Can you work these out from the model? Positions are in its coordinate system, mm. A direction names the side the tool comes from. Give positions to 0.01 mm unless a question says otherwise; leave off trailing zeros. Loops run counter-clockwise (first coordinate to the right, second up) from the corner with the lowest first, then second, coordinate; pieces in that order, holes last. Notation, with made-up numbers: (19.5, 38) -> (42.5, 38) arc R22 cw to (42.5, 69) -> close; hole circle Ø8 at (-11, 56). An arc over 180 degrees is marked (long way). Return JSON: item names as keys, results as strings. Group by question number.
Q1. Will these pins go through, and if not, where does the flat tip stop? pin 1 (0.6 mm diameter, centred on y = -11, z = 4, fed in from -X); pin 2 (0.6 mm diameter, centred on y = -11, z = 11, fed in from +X).
Q2. Suppose I cut it at A-A, the plane z = 6.5. Please give me the cut outline in (x, y), and give its area (3 significant figures).
Q3. Which directions (+Z, -Z, +X, -X, +Y, -Y) give clear straight access to the entire face, cutting with the end or side of a thin tool? Please do faces 1 (the flat face through (-11.498, -11, 7)), 2 (the flat face through (-5, -10, 8)), 3 (the flat face through (-1.4, 25, 7.4)).
Q4. I need wall thicknesses on line 1 along Y through (x, z) = (-15.75, 8.25); line 2 along Y through (x, z) = (-11.75, 10.75); line 3 along X through (y, z) = (8, 1). Which ranges of each line are inside material? Lowest first, please. Write a range as [from, to].
```python
from build123d import *

# Parameters (mm, degrees)
F0_W         = 20
F0_H         = 15
F1_DEPTH     = 10
F2_R         = 1
F4_DEPTH     = 15
F5_T1_DEPTH  = 30
F5_T3_DEPTH  = 8.75
F5_T6_ANGLE  = 80.7474763736
F5_T8_ANGLE  = 80.7474763736
F6_R         = 1
F7_T1_DEPTH  = 13
F7_S5_W      = 1
F7_S5_H      = 1
F7_T6_DEPTH  = 1
F7_S11_W     = 1
F7_S11_H     = 1
F7_T12_DEPTH = 1
F9_DEPTH     = 15


# Not quite as in the source:
# - a fillet or chamfer that OpenCascade refuses, or shapes differently, is made with other operations: its cross-section is extruded or revolved along the edge and cut away or added


with BuildPart() as f1:
    # F0 (on Front) → F1 (new body)
    with BuildSketch(Plane.XZ):
        with Locations((-10, 7.5)):
            Rectangle(F0_W, F0_H)
    extrude(amount=F1_DEPTH)

    # F2
    f2_edges = [f1.edges().sort_by_distance(p)[0] for p in [
        (-20, -5, 15),
        (0, -5, 15),
        (-20, -5, 0),
        (0, -5, 0),
    ]]
    fillet(f2_edges, radius=F2_R)

    # F3 (on Top) → F4 (join)
    with BuildSketch(Plane.XY):
        with BuildLine():
            Line((-20, 0), (0, 0))
            Line((0, 0), (0, 25))
            Line((0, 25), (-2, 25))
            ThreePointArc((-2, 25), (-15.0318358344, 15.4029218007), (-20, 0))
        make_face()
    extrude(amount=F4_DEPTH)

    # F5: fillet of radius 1 on 6 edges, made by hand

    # F5_s2 → F5_t1 (cut)
    with BuildSketch(Plane.XZ.offset(-27.5)):
        with BuildLine():
            ThreePointArc((-1, 15), (-0.2928932188, 14.7071067812), (0, 14))
            Line((0, 14), (0, 15))
            Line((0, 15), (-1, 15))
        make_face()
        with BuildLine():
            ThreePointArc((-1, 0), (-0.2928932188, 0.2928932188), (0, 1))
            Line((0, 1), (0, 0))
            Line((0, 0), (-1, 0))
        make_face()
    extrude(amount=F5_T1_DEPTH, mode=Mode.SUBTRACT)

    # F5_s4 → F5_t3 (cut)
    with BuildSketch(Plane.YZ.offset(-6.25)):
        with BuildLine():
            ThreePointArc((25, 14), (24.7071067812, 14.7071067812), (24, 15))
            Line((24, 15), (25, 15))
            Line((25, 15), (25, 14))
        make_face()
        with BuildLine():
            ThreePointArc((25, 1), (24.7071067812, 0.2928932188), (24, 0))
            Line((24, 0), (25, 0))
            Line((25, 0), (25, 1))
        make_face()
    extrude(amount=F5_T3_DEPTH, mode=Mode.SUBTRACT)

    # F5_s5 → F5_t6 (revolve, cut)
    with BuildSketch(Plane(origin=(6.1966627118, 1.0094707841, 0), x_dir=(0, 0, 1), z_dir=(0.9869892856, 0.1607860383, 0))):
        with BuildLine():
            ThreePointArc((14, -25.3383332565), (14.7071067812, -25.0454400377), (15, -24.3383332565))
            Line((15, -24.3383332565), (15, -25.3383332565))
            Line((15, -25.3383332565), (14, -25.3383332565))
        make_face()
    revolve(axis=Axis((6.3611111111, 0, 15), (0, 0, 1)), revolution_arc=F5_T6_ANGLE, mode=Mode.SUBTRACT)

    # F5_s7 → F5_t8 (revolve, cut)
    with BuildSketch(Plane(origin=(6.1966627118, 1.0094707841, 0), x_dir=(0, 0, 1), z_dir=(0.9869892856, 0.1607860383, 0))):
        with BuildLine():
            ThreePointArc((1, -25.3383332565), (0.2928932188, -25.0454400377), (0, -24.3383332565))
            Line((0, -24.3383332565), (0, -25.3383332565))
            Line((0, -25.3383332565), (1, -25.3383332565))
        make_face()
    revolve(axis=Axis((6.3611111111, 0, 0), (0, 0, 1)), revolution_arc=F5_T8_ANGLE, mode=Mode.SUBTRACT)

    # F6
    f6_edges = [f1.edges().sort_by_distance(p)[0] for p in [
        (-2, 25, 7.5),
    ]]
    fillet(f6_edges, radius=F6_R)

    # F7: fillet of radius 1 on 1 edges, made by hand

    # F7_s2 → F7_t1 (cut)
    with BuildSketch(Plane.XY.offset(1)):
        with BuildLine():
            ThreePointArc((-1, 25), (-0.2928932188, 24.7071067812), (0, 24))
            Line((0, 24), (0, 25))
            Line((0, 25), (-1, 25))
        make_face()
    extrude(amount=F7_T1_DEPTH, mode=Mode.SUBTRACT)


with BuildPart() as f7_tool4:
    # F7_s5 → F7_t6 (new body)
    with BuildSketch(Plane.XZ.offset(-24)):
        with Locations((-0.5, 0.5)):
            Rectangle(F7_S5_W, F7_S5_H)
    extrude(amount=-F7_T6_DEPTH)

    # F7_s7 → F7_t8 (revolve, cut)
    with BuildSketch(Plane(origin=(-1, 24, 1), x_dir=(-0.7071067812, 0, 0.7071067812), z_dir=(-0.7071067812, 0, -0.7071067812))):
        with BuildLine():
            ThreePointArc((0, -1), (1, 0), (0, 1))
            Line((0, 1), (0, -1))
        make_face()
    revolve(axis=Axis((-1, 24, 1), (0, 1, 0)), mode=Mode.SUBTRACT)


with BuildPart() as f1_1:
    add(f1.part)

    # F7_t3: cut F7_tool4
    add(f7_tool4.part, mode=Mode.SUBTRACT)


with BuildPart() as f7_tool10:
    # F7_s11 → F7_t12 (new body)
    with BuildSketch(Plane.XZ.offset(-24)):
        with Locations((-0.5, 14.5)):
            Rectangle(F7_S11_W, F7_S11_H)
    extrude(amount=-F7_T12_DEPTH)

    # F7_s13 → F7_t14 (revolve, cut)
    with BuildSketch(Plane(origin=(-1, 24, 14), x_dir=(-0.7071067812, 0, -0.7071067812), z_dir=(0.7071067812, 0, -0.7071067812))):
        with BuildLine():
            ThreePointArc((0, -1), (1, 0), (0, 1))
            Line((0, 1), (0, -1))
        make_face()
    revolve(axis=Axis((-1, 24, 14), (0, 1, 0)), mode=Mode.SUBTRACT)


with BuildPart() as f1_2:
    add(f1_1.part)

    # F7_t9: cut F7_tool10
    add(f7_tool10.part, mode=Mode.SUBTRACT)

    # F8 (on Top) → F9 (join, through all)
    with BuildSketch(Plane.XY):
        with BuildLine():
            Line((-9, -10), (-11.4979991994, -10))
            Line((-11.4979991994, -10), (-11.4979991994, -12))
            ThreePointArc((-11.4979991994, -12), (-10.2489995997, -10.8), (-9, -12))
            Line((-9, -12), (-9, -10))
        make_face()
    extrude(amount=F9_DEPTH)


solid = f1_2.part
```
Ans:
{
 "1": {"pin 1": "stops at x = -11.5", "pin 2": "stops at x = -9"},
 "2": {"outline": "(-20, -10) -> (-11.5, -10) -> (-11.5, -12) arc R1.25 cw to (-9, -12) -> (-9, -10) -> (0, -10) -> (0, 24) arc R1 ccw to (-1, 25) -> (-1.84, 25) arc R1 ccw to (-2.16, 24.95) arc R26.36 ccw to (-20, 0) -> close", "area": "582 mm^2"},
 "3": {"face 1": "+Z, -Z, -X, -Y", "face 2": "+Z, -Z, +X, -Y", "face 3": "+Z, -Z, +X, -X, +Y"},
 "4": {"line 1": "y = [-10, 14.35]", "line 2": "y = [-10, 19.15]", "line 3": "x = [-18.76, 0]"}
}
